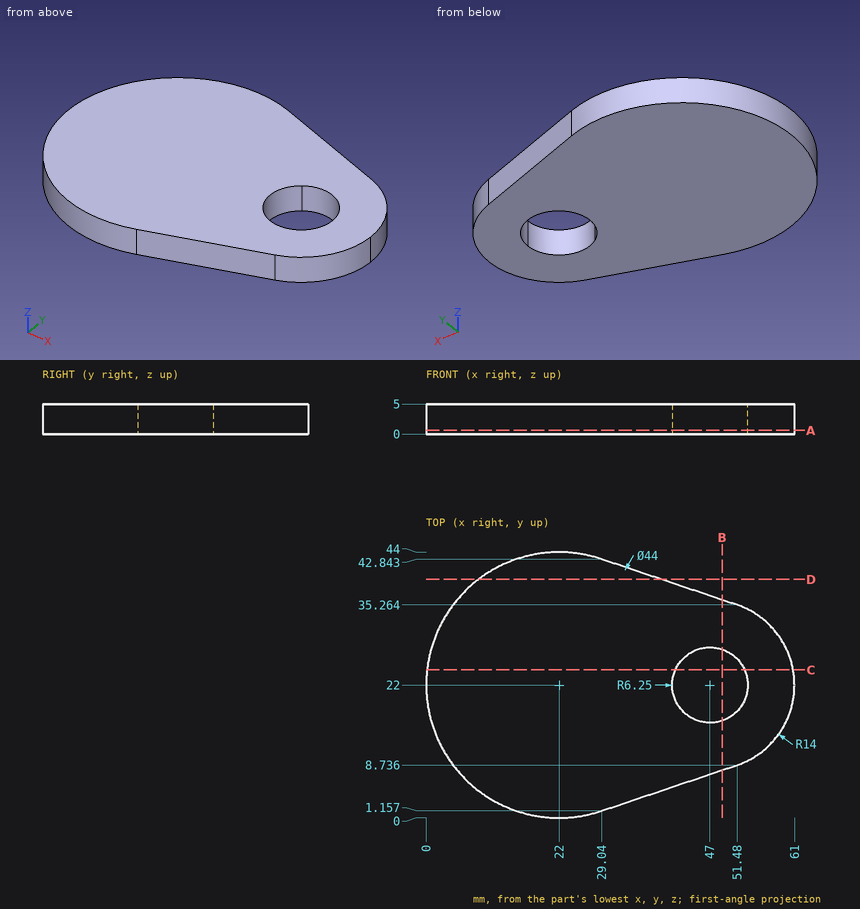
Can you work these out from the drawing? Everything is in mm from the part's minimum corner. Give positions to 0.01 mm unless a question says otherwise; leave off trailing zeros. Order: outer loops, then holes, each group sorted by start corner. A loop starts at its lowest first (then second) coordinate and runs counter-clockwise, first axis right, second up. Notation, with made-up numbers: (67.25, -34.75) -> (86.25, -34.75) arc R27 ccw to (86.25, 4.25) -> close; hole circle Ø4 at (75, 25.25). An arc over 180 degrees is marked (long way). Return JSON: item names as keys, results as strings.
1. Imagine slicing it at C-C on y = 24.5. List the corners of the cut face in (x, z) for me (1 decimal).
Answer list:
{"outline": "(0.1, 0) -> (41.3, 0) -> (41.3, 5) -> (0.1, 5) -> close; (52.7, 0) -> (60.8, 0) -> (60.8, 5) -> (52.7, 5) -> close"}
2. Imagine slicing it at A-A on z = 0.65. List the corners of the cut face in (x, y) for me.
Answer list:
{"outline": "(29.04, 1.16) -> (51.48, 8.74) arc R14 ccw to (51.48, 35.26) -> (29.04, 42.84) arc R22 ccw (long way) to start; hole circle Ø12.5 at (47, 22)"}
3. Imagine slicing it at D-D on y = 39.5. List the corners of the cut face in (x, z) for me.
Answer list:
{"outline": "(8.67, 0) -> (38.94, 0) -> (38.94, 5) -> (8.67, 5) -> close"}
4. For pin 1 Ø1 at (x, y) = (39.5, 29.5) entering from -Z; pin 2 Ø1 at (y, z) = (21.5, 3) entering from -X; pin 3 Ø1 at (y, z) = (28.5, 4) entering from +X; pin 4 Ø2 at (y, z) = (17, 1) entering from -X, each with a flat end and sliding along its axis, tell me the tip position at first contact or that it passes through.
Answer list:
{"pin 1": "stops at z = 0", "pin 2": "stops at x = 0", "pin 3": "stops at x = 59.65", "pin 4": "stops at x = 0.37"}
5. I need wall thicknesses on line 1 (Y direction, x = 15, z = 4.4); line 2 (X direction, y = 17.5, z = 1.6) (1 decimal); line 3 (Y direction, x = 45.5, z = 3.85). Which ranges of each line are inside material? Lowest first, please. Write a range as from..to.
Answer list:
{"line 1": "y = 1.14..42.86", "line 2": "x = 0.5..42.7, 51.3..60.3", "line 3": "y = 6.72..15.93, 28.07..37.28"}
6. Imagine slicing it at B-B on x = 49. List the corners of the cut face in (y, z) for me, then the cut area to 3 significant figures.
Answer list:
{"outline": "(7.9, 0) -> (16.08, 0) -> (16.08, 5) -> (7.9, 5) -> close; (27.92, 0) -> (36.1, 0) -> (36.1, 5) -> (27.92, 5) -> close", "area": "81.8 mm2"}
